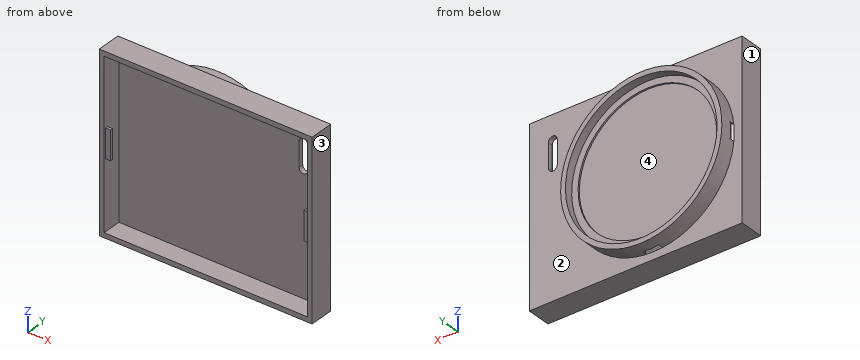
```python
from build123d import *

# Parameters (mm, degrees)
SKETCH1_W            = 132
SKETCH1_H            = 109
BOSS_EXTRUDE1_DEPTH  = 15
SKETCH2_W            = 126
SKETCH2_H            = 103
CUT_EXTRUDE1_DEPTH   = 12
SKETCH3_W            = 18
SKETCH3_H            = 1.5
BOSS_EXTRUDE6_DEPTH  = 3
SKETCH6_W            = 18
SKETCH6_H            = 1.5
BOSS_EXTRUDE7_DEPTH  = 3
CUT_EXTRUDE2_DEPTH   = 10
SKETCH13_R           = 50
BOSS_EXTRUDE10_DEPTH = 4
SKETCH18_R           = 47
CUT_EXTRUDE6_DEPTH   = 3
SKETCH19_R           = 50
BOSS_EXTRUDE11_DEPTH = 6
SKETCH20_R           = 47
CUT_EXTRUDE7_DEPTH   = 5
SKETCH21_R           = 43
CUT_EXTRUDE8_DEPTH   = 3
SKETCH22_W           = 10
SKETCH22_H           = 2
CUT_EXTRUDE10_DEPTH  = 8.2
CHAMFER2_SIZE        = 1.3
CHAMFER2_SIZE2       = 0.9102698
FILLET2_R            = 1
SKETCH23_W           = 10
SKETCH23_H           = 2
CUT_EXTRUDE11_DEPTH  = 8.2
CHAMFER3_SIZE        = 1
CHAMFER3_SIZE2       = 0.869286738
FILLET3_R            = 1
SKETCH24_W           = 10
SKETCH24_H           = 2
CUT_EXTRUDE12_DEPTH  = 8.2
CHAMFER4_SIZE        = 1
CHAMFER4_SIZE2       = 0.869286738
FILLET4_R            = 1


with BuildPart() as part:
    # Sketch1 → Boss-Extrude1 (new body)
    with BuildSketch(Plane(origin=(0, 0, 0), x_dir=(1, 0, 0), z_dir=(0, 1, 0))):
        Rectangle(SKETCH1_W, SKETCH1_H)
    extrude(amount=BOSS_EXTRUDE1_DEPTH)

    # Sketch2 → Cut-Extrude1 (cut)
    with BuildSketch(Plane.XZ):
        Rectangle(SKETCH2_W, SKETCH2_H)
    extrude(amount=-CUT_EXTRUDE1_DEPTH, mode=Mode.SUBTRACT)

    # Sketch3 → Boss-Extrude6 (add)
    with BuildSketch(Plane(origin=(-63, 0, 0), x_dir=(0, 0, -1), z_dir=(1, 0, 0))):
        with Locations((0, 2)):
            Rectangle(SKETCH3_W, SKETCH3_H)
    extrude(amount=BOSS_EXTRUDE6_DEPTH)

    # Sketch6 → Boss-Extrude7 (add)
    with BuildSketch(Plane.ZY.offset(-63)):
        with Locations((0, 2)):
            Rectangle(SKETCH6_W, SKETCH6_H)
    extrude(amount=BOSS_EXTRUDE7_DEPTH)

    # Sketch14 → Cut-Extrude2 (cut)
    with BuildSketch(Plane(origin=(0, 15, 0), x_dir=(1, 0, 0), z_dir=(0, 1, 0))):
        with BuildLine():
            Line((48.646447832, -24.177866046), (48.646447832, -39.177866046))
            ThreePointArc((48.646447832, -39.177866046), (51.396447832, -41.927866046), (54.146447832, -39.177866046))
            Line((54.146447832, -39.177866046), (54.146447832, -24.177866046))
            ThreePointArc((54.146447832, -24.177866046), (51.396447832, -21.427866046), (48.646447832, -24.177866046))
        make_face()
    extrude(amount=-CUT_EXTRUDE2_DEPTH, mode=Mode.SUBTRACT)

    # Sketch13 → Boss-Extrude10 (add)
    with BuildSketch(Plane(origin=(0, 15, 0), x_dir=(1, 0, 0), z_dir=(0, 1, 0))):
        with Locations(Location((-11.133590864, 0, 0), (0, 0, 90))):
            Circle(SKETCH13_R)
    extrude(amount=BOSS_EXTRUDE10_DEPTH)

    # Sketch18 → Cut-Extrude6 (cut)
    with BuildSketch(Plane(origin=(0, 19, 0), x_dir=(1, 0, 0), z_dir=(0, 1, 0))):
        with Locations(Location((-11.133590864, 0, 0), (0, 0, 270))):
            Circle(SKETCH18_R)
    extrude(amount=-CUT_EXTRUDE6_DEPTH, mode=Mode.SUBTRACT)

    # Sketch19 → Boss-Extrude11 (add)
    with BuildSketch(Plane(origin=(0, 19, 0), x_dir=(1, 0, 0), z_dir=(0, 1, 0))):
        with Locations(Location((-11.133590864, 0, 0), (0, 0, 90))):
            Circle(SKETCH19_R)
    extrude(amount=BOSS_EXTRUDE11_DEPTH)

    # Sketch20 → Cut-Extrude7 (cut)
    with BuildSketch(Plane(origin=(0, 25, 0), x_dir=(1, 0, 0), z_dir=(0, 1, 0))):
        with Locations(Location((-11.133590864, 0, 0), (0, 0, 270))):
            Circle(SKETCH20_R)
    extrude(amount=-CUT_EXTRUDE7_DEPTH, mode=Mode.SUBTRACT)

    # Sketch21 → Cut-Extrude8 (cut)
    with BuildSketch(Plane(origin=(0, 20, 0), x_dir=(1, 0, 0), z_dir=(0, 1, 0))):
        with Locations(Location((-11.133590864, 0, 0), (0, 0, 270))):
            Circle(SKETCH21_R)
    extrude(amount=-CUT_EXTRUDE8_DEPTH, mode=Mode.SUBTRACT)

    # Sketch22 → Cut-Extrude10 (cut)
    with BuildSketch(Plane.ZY.offset(66)):
        with Locations((0, 16.991930037)):
            Rectangle(SKETCH22_W, SKETCH22_H)
    extrude(amount=-CUT_EXTRUDE10_DEPTH, mode=Mode.SUBTRACT)

    # Chamfer2
    chamfer2_edges = [part.edges().sort_by_distance(p)[0] for p in [
        (-61.133590864, 15.991930037, 0),
    ]]
    chamfer2_side = [part.faces().sort_by_distance(p)[0] for p in [
        (-59.42592439, 15.991930037, 0),
    ]]
    chamfer(chamfer2_edges, length=CHAMFER2_SIZE, length2=CHAMFER2_SIZE2, reference=chamfer2_side[0])

    # Fillet2
    fillet2_edges = [part.edges().sort_by_distance(p)[0] for p in [
        (-59.833590864, 15.991930037, 0),
    ]]
    fillet(fillet2_edges, radius=FILLET2_R)

    # Sketch23 → Cut-Extrude11 (cut)
    with BuildSketch(Plane(origin=(0, 0, -54.5), x_dir=(-1, 0, 0), z_dir=(0, 0, -1))):
        with Locations((11.721254149, 17)):
            Rectangle(SKETCH23_W, SKETCH23_H)
    extrude(amount=-CUT_EXTRUDE11_DEPTH, mode=Mode.SUBTRACT)

    # Chamfer3
    chamfer3_edges = [part.edges().sort_by_distance(p)[0] for p in [
        (-13.931807962, 16, -49.921638405),
    ]]
    chamfer3_side = [part.faces().sort_by_distance(p)[0] for p in [
        (-11.119691984, 16, -0.208830113),
    ]]
    chamfer(chamfer3_edges, length=CHAMFER3_SIZE, length2=CHAMFER3_SIZE2, reference=chamfer3_side[0])

    # Fillet3
    fillet3_edges = [part.edges().sort_by_distance(p)[0] for p in [
        (-11.724338174, 16, -48.996438826),
    ]]
    fillet(fillet3_edges, radius=FILLET3_R)

    # Sketch24 → Cut-Extrude12 (cut)
    with BuildSketch(Plane.XY.offset(54.5)):
        with Locations((-11.559090934, 17)):
            Rectangle(SKETCH24_W, SKETCH24_H)
    extrude(amount=-CUT_EXTRUDE12_DEPTH, mode=Mode.SUBTRACT)

    # Chamfer4
    chamfer4_edges = [part.edges().sort_by_distance(p)[0] for p in [
        (-11.561234683, 16, 49.998171174),
    ]]
    chamfer4_side = [part.faces().sort_by_distance(p)[0] for p in [
        (-11.120399941, 16, 0.097012581),
    ]]
    chamfer(chamfer4_edges, length=CHAMFER4_SIZE, length2=CHAMFER4_SIZE2, reference=chamfer4_side[0])

    # Fillet4
    fillet4_edges = [part.edges().sort_by_distance(p)[0] for p in [
        (-11.56132378, 16, 48.998133072),
    ]]
    fillet(fillet4_edges, radius=FILLET4_R)


solid = part.part
```
Design review of the part built by this model. Coordinates are the model's own, in mm. Face numbers are marked on the shaded views. Round coordinates to 2 decimals unless told otherwise and drop trailing zeros. Write each loop counter-clockwise with the first axis right and the second up, starting at its lowest first coordinate (ties: lowest second). Pieces come first, ordered by that corner, then holes.
Item 1: We need section A-A on y = 10.5. Write out the cut boundary in (x, z).
Item 2: For probe 1 along X at (y, z) = (19.45, 0); probe 2 along Z at (x, y) = (-16, 1.75); probe 3 along X at (y, z) = (21.1, 0), list the stretches that pass through material, from the lowest coordinate up.
Item 3: We need section C-C on z = -15.5. Write out the cut boundary in (x, y), and give its area (3 significant figures).
Item 4: Clearance check with flat-ended pins moving along their axes: pin 1 Ø2.5 at (x, z) = (-13.5, -48) entering from -Y; pin 2 Ø3.5 at (x, z) = (-59.5, 0.5) entering from -Y; pin 3 Ø2 at (y, z) = (21.5, 18.5) entering from +X. State where each tip first meets the part, or that it passes through.
Item 5: The part is to be moulded in two halves that separate along X. For the marked faces 1, 2, 3 and 4, say which applies: +X half, -X half, draft (parallel to the pull), parting line (faces both ways), or undercut.
Item 6: We need section B-B on x = -37. Write out the cut boundary in (y, z).
Returned:
1. outline: (-66, -54.5) - (66, -54.5) - (66, 54.5) - (-66, 54.5) - close; hole (-63, -51.5) - (63, -51.5) - (63, 51.5) - (-63, 51.5) - close
2. probe 1: x = -61.13 to -54.13, 31.87 to 38.87
2. probe 2: z = -54.5 to -51.5, 51.5 to 54.5
2. probe 3: x = -61.13 to -58.13, 35.87 to 38.87
3. outline: (-66, 0) - (-63, 0) - (-63, 12) - (63, 12) - (63, 0) - (66, 0) - (66, 15) - (36.4, 15) - (36.4, 25) - (33.24, 25) - (33.24, 20) - (28.98, 20) - (28.98, 19) - (33.24, 19) - (33.24, 16) - (-55.5, 16) - (-55.5, 19) - (-51.24, 19) - (-51.24, 20) - (-55.5, 20) - (-55.5, 25) - (-58.67, 25) - (-58.67, 15) - (-66, 15) - close
3. area: 629 mm2
4. pin 1: stops at y = 12
4. pin 2: stops at y = 1.25
4. pin 3: stops at x = 35.7
5. face 1: -X half
5. face 2: draft
5. face 3: +X half
5. face 4: undercut
6. outline: (0, -54.5) - (15, -54.5) - (15, -42.79) - (25, -42.79) - (25, -39.24) - (20, -39.24) - (20, -34.35) - (19, -34.35) - (19, -39.24) - (16, -39.24) - (16, 39.24) - (19, 39.24) - (19, 34.35) - (20, 34.35) - (20, 39.24) - (25, 39.24) - (25, 42.79) - (15, 42.79) - (15, 54.5) - (0, 54.5) - (0, 51.5) - (12, 51.5) - (12, -51.5) - (0, -51.5) - close
